Geometry: final body of the model. Coordinates: model frame, mm. Face numbers are marked on the shaded views. A direction names the side the tool comes from. Round coordinates to 2 decimals unless told otherwise and drop trailing zeros. Loops run counter-clockwise (first coordinate to the right, second up) from the corner with the lowest first, then second, coordinate; pieces in that order, holes last. Notation, with made-up numbers: (-8, 59) - (-1, 59) arc R28 cw to (-1, 97) - close; hole circle Ø6 at (27, 1.5). An arc over 180 degrees is marked (long way). Return JSON: item names as keys, results as strings. Group by question number.
1. Section B-B on x = 4.75. Return loops of the section in (y, z).
2. Draft query along Z for the marked faces 4, 5 and 6. Return one class per face: +Z half, -Z half, draft (parallel to the pull), parting line (faces both ways), or undercut.
3. Set-up query: the marked faces 1, 2 and 3. Return all of +Z, -Z, +X, -X, +Y, -Y with unobstructed straight access to the full face (end or side cutting, diameter ignored); none if empty.
4. Material intervals for probe 1 along X at (y, z) = (1, -3); probe 2 along Z at (x, y) = (6.25, -1); probe 3 along Z at (x, y) = (1.25, -1.25), sorted ascending.
5. First-contact query: pin 1 Ø2 at (x, y) = (2, 0) entering from -Z; pin 2 Ø1.5 at (x, y) = (0, 1) entering from -Z. Flat tips, straight axial feed; report the tip coordinate or a pass-through.
from build123d import *

# Parameters (mm, degrees)
CUT_EXTRUDE1_DEPTH = 2


with BuildPart() as part:
    # Sketch1 → Revolve1 (revolve)
    with BuildSketch(Plane.XY, mode=Mode.PRIVATE) as revolve1_sk:
        with BuildLine():
            Line((11.7465, 2), (0.2, 2))
            ThreePointArc((0.2, 2), (0.058578644, 2.058578644), (0, 2.2))
            Line((0, 2.2), (0, 3.5))
            Line((0, 3.5), (-3.8, 3.5))
            ThreePointArc((-3.8, 3.5), (-3.941421356, 3.441421356), (-4, 3.3))
            Line((-4, 3.3), (-4, 0))
            Line((-4, 0), (12, 0))
            Line((12, 0), (12, 1.7465))
            Line((12, 1.7465), (11.7465, 2))
        make_face()
    revolve(revolve1_sk.sketch.rotate(Axis((-4, 0, 0), (1, 0, 0)), 90), axis=Axis((-4, 0, 0), (1, 0, 0)))

    # Sketch2 → Cut-Extrude1 (cut)
    with BuildSketch(Plane.ZY.offset(4)):
        Polygon((1.535, 0.886232663), (0, 1.772465326), (-1.535, 0.886232663), (-1.535, -0.886232663), (0, -1.772465326), (1.535, -0.886232663), align=None)
    extrude(amount=-CUT_EXTRUDE1_DEPTH, mode=Mode.SUBTRACT)


solid = part.part
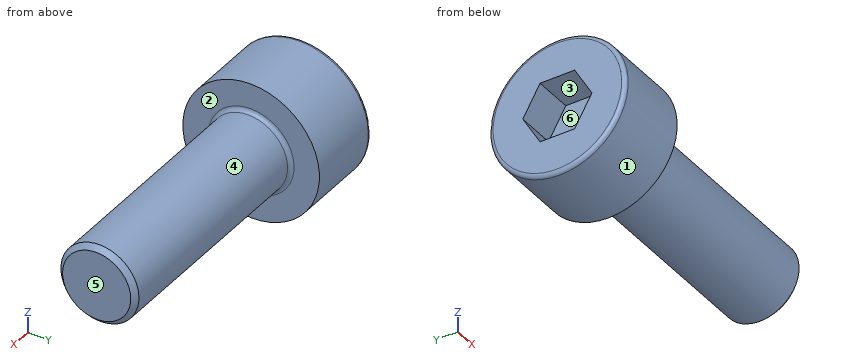
Taken from the geometry:
{
 "1": {"outline": "circle Ø4 at (0, 0)"},
 "2": {"face 4": "parting line", "face 5": "draft", "face 6": "undercut"},
 "3": {"face 1": "+X, -X", "face 2": "+X", "face 3": "-X"},
 "4": {"probe 1": "-4 to 0", "probe 2": "-1.73 to 1.73", "probe 3": "-1.56 to 1.56"},
 "5": {"pin 1": "z = -2", "pin 2": "z = -3.49"}
}
